For this review, use the dimensioned drawing (mm, ordinates from the lowest corner) and the shaded views. A direction names the side the tool comes from. Give positions to 0.01 mm unless a question says otherwise; leave off trailing zeros. Loops run counter-clockwise (first coordinate to the right, second up) from the corner with the lowest first, then second, coordinate; pieces in that order, holes last. Notation, with made-up numbers: (64, -16) -> (108, -16) arc R17 ccw to (108, -1) -> close; hole circle Ø1 at (39.25, -31.5). An arc over 180 degrees is marked (long way). Use a Markdown table: item, result. Add a question column.
1. Add section B-B (x = 20.5). State the section outline as (y, z) points.
2. Draft analysis for pull direction X (two halves, no side actions). For the marked faces 3, 4 and 5, state which applies: pulls with the +X half, pulls with the -X half, needs draft (parallel to the pull), parting line crosses it, or undercut.
3. To check wall thickness, follow line 1 (Z direction, x = 53, y = 0.9); line 2 (Z direction, x = 69.9, y = 1.4); line 3 (X direction, y = 1, z = 12). State the ranges of each line that lie inside material, in increasing order.
4. For the marked faces 1 and 2, list the 3-axis set-ups (+Z, -Z, +X, -X, +Y, -Y) from which the entire face can be reached by the end or side of a thin tool; tool diameter is ignored.
5. Add section A-A (z = 75.5). State the section outline as (x, y) points.
6. Add section D-D (x = 53). State the section outline as (y, z) points.
7. For pin 1 Ø0.8 at (x, y) = (41, 29.5) entering from -Z; pin 2 Ø6 at (x, z) = (23.5, 69.5) entering from -Y; pin 3 Ø2 at (x, y) = (104.5, 16.5) entering from -Z (1 decimal), all flat-tipped, find the tip position at first contact; note any pin that passes through.
8. Add section C-C (z = 63.5). State the section outline as (x, y) points.
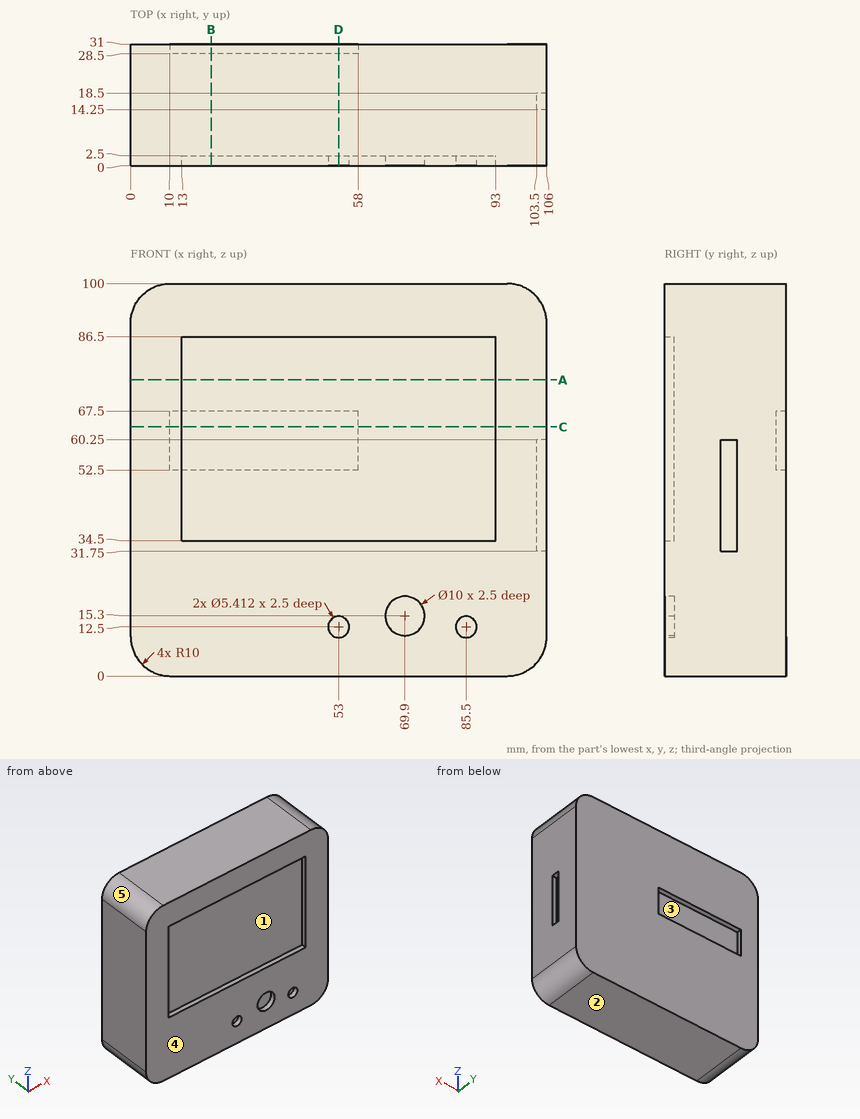
Taken from the geometry:
| question | item | result |
|---|---|---|
| 1 | outline | (0, 0) -> (31, 0) -> (31, 52.5) -> (28.5, 52.5) -> (28.5, 67.5) -> (31, 67.5) -> (31, 100) -> (0, 100) -> (0, 86.5) -> (2.5, 86.5) -> (2.5, 34.5) -> (0, 34.5) -> close |
| 2 | face 3 | undercut |
| 2 | face 4 | needs draft |
| 2 | face 5 | pulls with the -X half |
| 3 | line 1 | z = 0 to 9.79, 15.21 to 34.5, 86.5 to 100 |
| 3 | line 2 | z = 0 to 10.3, 20.3 to 34.5, 86.5 to 100 |
| 3 | line 3 | x = 0 to 50.34, 55.66 to 66.14, 73.66 to 82.84, 88.16 to 106 |
| 4 | face 1 | -Y |
| 4 | face 2 | -Z, +X, -X, +Y, -Y |
| 5 | outline | (0, 0) -> (13, 0) -> (13, 2.5) -> (93, 2.5) -> (93, 0) -> (106, 0) -> (106, 31) -> (0, 31) -> close |
| 6 | outline | (0, 0) -> (31, 0) -> (31, 52.5) -> (28.5, 52.5) -> (28.5, 67.5) -> (31, 67.5) -> (31, 100) -> (0, 100) -> (0, 86.5) -> (2.5, 86.5) -> (2.5, 34.5) -> (0, 34.5) -> (0, 15.21) -> (2.5, 15.21) -> (2.5, 9.79) -> (0, 9.79) -> close |
| 7 | pin 1 | stops at z = 0 |
| 7 | pin 2 | stops at y = 2.5 |
| 7 | pin 3 | stops at z = 3.4 |
| 8 | outline | (0, 0) -> (13, 0) -> (13, 2.5) -> (93, 2.5) -> (93, 0) -> (106, 0) -> (106, 31) -> (58, 31) -> (58, 28.5) -> (10, 28.5) -> (10, 31) -> (0, 31) -> close |
